```python
from build123d import *

# Parameters (mm, degrees)
BOSS_EXTRUDE1_DEPTH = 3.175


with BuildPart() as part:
    # Sketch1 → Boss-Extrude1 (new body)
    with BuildSketch(Plane(origin=(0, 0, 0), x_dir=(1, 0, 0), z_dir=(0, 1, 0))):
        with BuildLine():
            Line((-4.202954503, 19.05), (-42.302954503, 19.05))
            Line((-42.302954503, 19.05), (-88.9, 12.7))
            Line((-88.9, 12.7), (-88.9, -12.7))
            Line((-88.9, -12.7), (-42.302954503, -19.05))
            Line((-42.302954503, -19.05), (-1.945497784, -19.05))
            ThreePointArc((-1.945497784, -19.05), (-0.010483672, 0.181529292), (-4.202954503, 19.05))
        make_face()
    extrude(amount=-BOSS_EXTRUDE1_DEPTH)


solid = part.part
```
Here's how the part is built. I have some questions about the finished solid (model axes, mm). Give positions to 0.01 mm unless a question says otherwise; leave off trailing zeros. Write each loop counter-clockwise with the first axis right and the second up, starting at its lowest first coordinate (ties: lowest second). Pieces come first, ordered by that corner, then holes. Notation, with made-up numbers: M 56.25,-35.5 L 64.25,-35.5 A26 ccw 64.25,-15.5 Z; hole C 77.25,-16.5 d9. An arc over 180 degrees is marked long. Put each result on its own line as item: value. Start each with the question number.
Item 1: If we section it at A-A, the plane y = -1.5: Write out the boundary of the cut face in (x, z), then the cut area to 3 significant figures.
Item 2: I need wall thicknesses on L1, parallel to X at y = -2.2, z = 0.5; L2, parallel to X at y = -0.6, z = -2.5; L3, parallel to Z at x = -71, y = -2.45. Which ranges of each line are inside material? Lowest first, please. Write a range as from..to.
Item 3: Will these pins go through, and if not, where does the flat tip stop? pin 1 (1 mm diameter, centred on y = -2, z = -7.5, fed in from +X); pin 2 (1 mm diameter, centred on x = -64, y = -1, fed in from -Z).
Item 4: If we section it at B-B, the plane z = 16.5: Write out the boundary of the cut face in (x, y) (3 decimals), then the cut area to 3 significant figures.
Item 5: If we section it at C-C, the plane x = -49: Write out the boundary of the cut face in (y, z) (3 decimals).
Values:
1. outline: M -88.9,-12.7 L -42.3,-19.05 L -4.2,-19.05 A60.86 ccw -1.95,19.05 L -42.3,19.05 L -88.9,12.7 Z
1. area: 3,050 mm²
2. L1: -88.9..0.03
2. L2: -88.9..-0.19
2. L3: -15.14..15.14
3. pin 1: x = -0.8
3. pin 2: z = -16.16
4. outline: M -61.015,-3.175 L -1.326,-3.175 L -1.326,0 L -61.015,0 Z
4. area: 190 mm²
5. outline: M -3.175,-18.137 L 0,-18.137 L 0,18.137 L -3.175,18.137 Z
